Design review of the part built by this model. Coordinates are the model's own, in mm. A direction names the side the tool comes from. Give positions to 0.01 mm unless a question says otherwise; leave off trailing zeros. Order: outer loops, then holes, each group sorted by start corner. A loop starts at its lowest first (then second) coordinate and runs counter-clockwise, first axis right, second up. Notation, with made-up numbers: (22, 5) -> (61, 5) arc R11 ccw to (61, 10) -> close; hole circle Ø2 at (85.25, 84). An arc over 180 degrees is marked (long way). Use a Markdown table: item, result. Add a question column.
```python
from build123d import *

# Parameters (mm, degrees)
SKETCH_1_W          = 34
SKETCH_1_H          = 30
SKETCH_1_R          = 2
EXTRUDE_1_DEPTH     = 17
EXTRUDE_3_REACH     = 41.002
SKETCH_4_R          = 8.07551033
CUT_EXTRUDE_1_DEPTH = 30


with BuildPart() as part:
    # 草图1 → 凸台-拉伸1 (new body)
    with BuildSketch(Plane(origin=(0, 0, 0), x_dir=(1, 0, 0), z_dir=(0, 1, 0))):
        with Locations((1.225705329, 2.956112853)):
            Rectangle(SKETCH_1_W, SKETCH_1_H)
        with Locations(Location((-10.774294671, 11.956112853, 0), (0, 0, 270))):
            Circle(SKETCH_1_R, mode=Mode.SUBTRACT)
        with Locations(Location((13.225705329, 11.956112853, 0), (0, 0, 90))):
            Circle(SKETCH_1_R, mode=Mode.SUBTRACT)
        with Locations(Location((13.225705329, -6.043887147, 0), (0, 0, 270))):
            Circle(SKETCH_1_R, mode=Mode.SUBTRACT)
        with Locations(Location((-10.774294671, -6.043887147, 0), (0, 0, 90))):
            Circle(SKETCH_1_R, mode=Mode.SUBTRACT)
    extrude(amount=EXTRUDE_1_DEPTH)

    # 凸台-拉伸3: up to this face of the body (flat: up to its plane)
    extrude_3_end = Plane(part.part.faces().sort_by_distance((1.225705329, 8.5, -17.956112853))[0])
    # 草图3 → 凸台-拉伸3 (add, up to the picked face)
    with BuildSketch(Plane.XY.offset(12.043887147), mode=Mode.PRIVATE) as extrude_3_sk1:
        Polygon((-4.926354977, 22), (-8.774294671, 17), (1.225705329, 17), (11.225705329, 17), (7.377765635, 22), align=None)
    extrude_3_tool1 = split(extrude(extrude_3_sk1.sketch, amount=-EXTRUDE_3_REACH, mode=Mode.PRIVATE), bisect_by=extrude_3_end, keep=Keep.BOTH, mode=Mode.PRIVATE)
    add(extrude_3_tool1.solids().sort_by(Axis((1.225705, 19.301473, 12.043887), (0, 0, -1)))[0])

    # 草图4 → 切除-拉伸1 (cut)
    with BuildSketch(Plane.XY.offset(12.043887147)):
        with Locations((1.225705329, 10.534716584)):
            Circle(SKETCH_4_R)
    extrude(amount=-CUT_EXTRUDE_1_DEPTH, mode=Mode.SUBTRACT)


solid = part.part
```
1) Insertion check: pin 1 (5 mm diameter, centred on x = -12, z = 2, fed in from +Y); pin 2 (6.5 mm diameter, centred on x = 13.23, z = -11.96, fed in from +Y); pin 3 (1.5 mm diameter, centred on y = 18, z = 7.5, fed in from -X). Each pin has a flat end and moves straight along its axis. Give the tip position at first contact, or say it passes through.
2) Add section A-A (z = 6.5). Give the boundary of the cut face in (x, y).
3) Add section B-B (y = 9.5). Give the boundary of the cut face in (x, z).
4) Add section C-C (x = -3.5). Give the boundary of the cut face in (y, z), then the cut area to 3 significant figures.
5) For L1, parallel to Z at x = 13.5, y = 4.5; L2, parallel to X at y = 3.5, z = 5.75; L3, parallel to Z at x = 15, y = 2.25, list the stretches that pass through material, from the lowest coordinate up. Write a range as [from, to].
6) Machinability: for faces 1 (the cylindrical face through (-12.126, 8.381, 7.518)), 2 (the flat face through (15, 17, -3)), 3 (the flat face through (-12, 17, -3)), which of the approach directions +Z, -Z, +X, -X, +Y, -Y give a long, thin tool a straight path to every point of the face, cutting with its end or side? Answer none if there is none.
7) The part is to be moulded in two halves that separate along X. For faces 4 (the cylindrical face through (-10.17, 8.38, -10.05)), 5 (the flat face through (9.3, 19.5, -2.7)), 6 (the flat face through (-6.82, 19.54, -2.75)), say which applies: +X half, -X half, draft (parallel to the pull), parting line (faces both ways), or undercut.
8) Add section D-D (x = 12.5). Give the boundary of the cut face in (y, z), then the cut area to 3 significant figures.
Worked answers:
| question | item | result |
|---|---|---|
| 1 | pin 1 | y = 17 |
| 1 | pin 2 | y = 18.62 |
| 1 | pin 3 | x = -8.58 |
| 2 | outline | (-15.77, 0) -> (-12.72, 0) -> (-12.72, 17) -> (-15.77, 17) -> close; (-8.83, 0) -> (11.28, 0) -> (11.28, 17) -> (11.23, 17) -> (7.38, 22) -> (-4.93, 22) -> (-8.77, 17) -> (-8.83, 17) -> close; (15.17, 0) -> (18.23, 0) -> (18.23, 17) -> (15.17, 17) -> close; hole circle Ø16.15 at (1.23, 10.53) |
| 3 | outline | (-15.77, -17.96) -> (-6.78, -17.96) -> (-6.78, 12.04) -> (-15.77, 12.04) -> close; (9.23, -17.96) -> (18.23, -17.96) -> (18.23, 12.04) -> (9.23, 12.04) -> close; hole circle Ø4 at (-10.77, -11.96); hole circle Ø4 at (-10.77, 6.04); hole circle Ø4 at (13.23, -11.96); hole circle Ø4 at (13.23, 6.04) |
| 4 | outline | (0, -17.96) -> (3.99, -17.96) -> (3.99, 12.04) -> (0, 12.04) -> close; (17.08, -17.96) -> (22, -17.96) -> (22, 12.04) -> (17.08, 12.04) -> close |
| 4 | area | 267 mm^2 |
| 5 | L1 | [-17.96, -13.94], [-9.98, 4.06], [8.02, 12.04] |
| 5 | L2 | [-15.77, -12.75], [-8.8, -2.74], [5.19, 11.25], [15.2, 18.23] |
| 5 | L3 | [-17.96, -12.88], [-11.03, 5.12], [6.97, 12.04] |
| 6 | face 1 | +Y, -Y |
| 6 | face 2 | +Z, -Z, +X, +Y |
| 6 | face 3 | +Z, -Z, -X, +Y |
| 7 | face 4 | undercut |
| 7 | face 5 | +X half |
| 7 | face 6 | -X half |
| 8 | outline | (0, -17.96) -> (17, -17.96) -> (17, -13.82) -> (0, -13.82) -> close; (0, -10.09) -> (17, -10.09) -> (17, 4.18) -> (0, 4.18) -> close; (0, 7.91) -> (17, 7.91) -> (17, 12.04) -> (0, 12.04) -> close |
| 8 | area | 383 mm^2 |
